Geometry: final body of the model. Coordinates: model frame, mm. Face numbers are marked on the shaded views. A direction names the side the tool comes from. Round coordinates to 2 decimals unless told otherwise and drop trailing zeros. Loops run counter-clockwise (first coordinate to the right, second up) from the corner with the lowest first, then second, coordinate; pieces in that order, holes last. Notation, with made-up numbers: (74, 15) - (129, 15) arc R21 ccw to (129, 36) - close; hole circle Ø4 at (-14, 67). An arc over 180 degrees is marked (long way). Return JSON: item names as keys, results as strings. Group by question number.
1. First-contact query: pin 1 Ø12.5 at (x, y) = (-45, 45) entering from +Z; pin 2 Ø14.5 at (x, y) = (45, 45) entering from -Z; pin 3 Ø10 at (x, y) = (-17.512, 6.5) entering from -Z; pin 4 Ø8 at (x, y) = (-18, 5.5) entering from +Z. Flat tips, straight axial feed; report the tip coordinate or a pass-through.
2. Section A-A on y = 45. Return loops of the section in (x, z), and give its area (3 significant figures).
3. Section D-D on y = 31. Return loops of the section in (x, z), and give its area (4 significant figures).
4. Material intervals for probe 1 along Y at (x, z) = (-42.5, -0.25); probe 2 along X at (y, z) = (-19, -1.5); probe 3 along X at (y, z) = (8.5, 1.25), sorted ascending.
5. Section B-B on z = 4.75. Count the separate pieces of the cut face and the enclosed holes in it, and give its area (3 significant figures).
6. Set-up query: the marked faces 1 and 2. Return all of +Z, -Z, +X, -X, +Y, -Y with unobstructed straight access to the full face (end or side cutting, diameter ignored); none if empty.
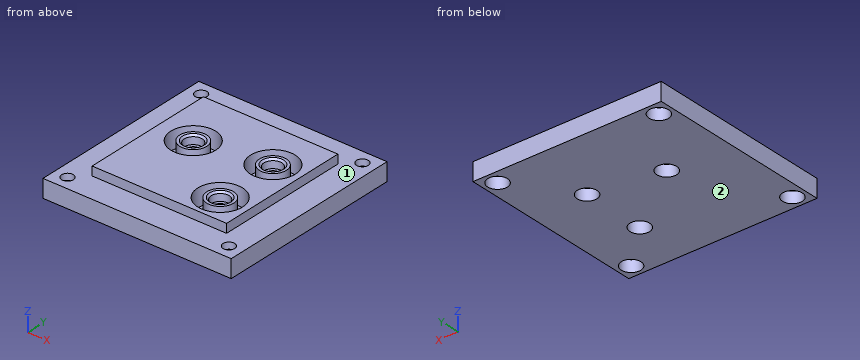
Autodesk Inventor part; units mm, degrees
ref_plane "YZ Plane" through (0, 0, 0) normal (1, 0, 0) x (0, 1, 0)
ref_plane "XZ Plane" through (0, 0, 0) normal (0, 1, 0) x (-1, 0, 0)
ref_plane "XY Plane" through (0, 0, 0) normal (0, 0, 1) x (1, 0, 0)
sketch "Skizze1" plane through (0, 0, 0) normal (0, 0, 1) x (1, 0, 0)
  line L0 (-52.5, 52.5) -> (52.5, 52.5)
  line L1 (52.5, 52.5) -> (52.5, -52.5)
  line L2 (52.5, -52.5) -> (-52.5, -52.5)
  line L3 (-52.5, -52.5) -> (-52.5, 52.5)
  line L4 (-52.5, 52.5) -> (52.5, -52.5) construction
  line L5 (52.5, 52.5) -> (-52.5, -52.5) construction
  point P0 (0, 0)
  dimension "d0" = 105
  dimension "d1" = 105
extrude "Extrusion1" add sketch "Skizze1" along normal mid plane 15
sketch "Skizze2" plane through (0, 0, -7.5) normal (0, 0, -1) x (-1, 0, 0)
  point P0 (0, 0)
  point P1 (17.512, 6.5)
  point P2 (-21.618, -22.607)
  point P3 (-21.618, 12.918)
  dimension "d4" = 21.618
  dimension "d5" = 22.607
  dimension "d6" = 12.918
  dimension "d8" = 17.512
  dimension "d16" = 6.5
hole "Bohrung1" at (21.618, -22.607, -7.5) at (21.618, 12.918, -7.5) at (-17.512, 6.5, -7.5) direction (0, 0, 1) diameter 6.6 end through all counterbore diameter 11 counterbore depth 6.4
sketch "Skizze4" plane through (0, 0, 7.5) normal (0, 0, 1) x (1, 0, 0)
  circle A0 centre (-17.512, 6.5) radius 3.3
  circle A1 centre (21.618, 12.918) radius 3.3
  circle A2 centre (21.618, -22.607) radius 3.3
  circle A3 centre (-17.512, 6.5) radius 5
  circle A4 centre (21.618, 12.918) radius 5
  circle A5 centre (21.618, -22.607) radius 5
  point P0 (0, 0)
  dimension "d24" = 10
  dimension "d25" = 10
  dimension "d26" = 10
extrude "Extrusion2" cut sketch "Skizze4" against normal blind 5 contours A0 | A1 | A2 | A3 | A4 | A5
chamfer "Fasen1" distance 1 angle 45 3 edges at (-22.512, 6.5, 7.5) (16.618, 12.918, 7.5) (16.618, -22.607, 7.5)
sketch "Skizze5" plane through (0, 0, 7.5) normal (0, 0, 1) x (1, 0, 0)
  line L0 (-37.5, 37.5) -> (37.5, 37.5)
  line L1 (37.5, 37.5) -> (37.5, -37.5)
  line L2 (37.5, -37.5) -> (-37.5, -37.5)
  line L3 (-37.5, -37.5) -> (-37.5, 37.5)
  line L4 (-37.5, 37.5) -> (37.5, -37.5) construction
  line L5 (37.5, 37.5) -> (-37.5, -37.5) construction
  line L6 (52.5, 52.5) -> (-52.5, 52.5)
  line L7 (52.5, -52.5) -> (52.5, 52.5)
  line L8 (-52.5, 52.5) -> (-52.5, -52.5)
  line L9 (-52.5, -52.5) -> (52.5, -52.5)
  point P0 (0, 0)
  dimension "d32" = 15
  dimension "d33" = 15
extrude "Extrusion3" cut sketch "Skizze5" against normal blind 5
sketch "Skizze6" plane through (0, 0, -7.5) normal (0, 0, -1) x (-1, 0, 0)
  line L0 (-52.5, -52.5) -> (52.5, -52.5)
  line L1 (52.5, -52.5) -> (52.5, 52.5)
  point P0 (0, 0)
  point P1 (45, -45)
  dimension "d36" = 7.5
  dimension "d37" = 7.5
hole "Bohrung2" at (-45, -45, -7.5) direction (0, 0, 1) diameter 6.6 end through all counterbore diameter 11 counterbore depth 6.4
pattern_circular "Runde Anordnung1" count 4 over 360 about axis through (0, 0, -10) along (0, 0, 1) of "Bohrung2"
sketch "Skizze7" plane through (0, 0, 7.5) normal (0, 0, 1) x (1, 0, 0)
  circle A0 centre (-17.512, 6.5) radius 3.3
  circle A1 centre (-17.512, 6.5) radius 7.5
  circle A2 centre (21.618, 12.918) radius 3.3
  circle A3 centre (21.618, 12.918) radius 7.5
  circle A4 centre (21.618, -22.607) radius 3.3
  circle A5 centre (21.618, -22.607) radius 7.5
  circle A6 centre (-17.512, 6.5) radius 12.5
  circle A7 centre (21.618, 12.918) radius 12.5
  circle A8 centre (21.618, -22.607) radius 5.5
  circle A9 centre (21.618, -22.607) radius 12.5
  point P0 (0, 0)
  dimension "d48" = 15
  dimension "d49" = 15
  dimension "d50" = 15
  dimension "d51" = 25
  dimension "d52" = 25
  dimension "d53" = 25
extrude "Extrusion4" cut sketch "Skizze7" against normal blind 10 contours A6 | A7 | A9
equation "\"d0\" = Breite_Magazin"
equation "\"d1\" = Tiefe_Magazin"
equation "\"d2\" = Hoehe_Bodenplatte"
equation "\"d27\" = Fuehrung_Tiefe"
equation "\"d29\" = Fase"
equation "\"d32\" = Wandstaerke"
equation "\"d33\" = Wandstaerke"
equation "\"d34\" = Fuehrung_Tiefe"
equation "\"d48\" = Feder_innen"
equation "\"d49\" = Feder_innen"
equation "\"d50\" = Feder_innen"
equation "\"d51\" = Feder_aussen"
equation "\"d52\" = Feder_aussen"
equation "\"d53\" = Feder_aussen"
equation "\"d54\" = Federfuehrung_Tiefe"
equation "\"Tiefe_Magazin\" = Breite_Magazin"
equation "\"Hoehe_Bodenplatte\" = 15"
equation "\"Fuehrung_Tiefe\" = 5"
equation "\"Fase\" = 1"
equation "\"Wandstaerke\" = 15"
equation "\"Feder_innen\" = 15"
equation "\"Feder_aussen\" = 25"
equation "\"Federfuehrung_Tiefe\" = 10"
properties part number "TS_Magazin_Grundplatte"
Taken from the geometry:
{
 "1": {"pin 1": "z = 2.5", "pin 2": "z = -7.5", "pin 3": "z = -1.1", "pin 4": "z = 6.61"},
 "2": {"outline": "(-52.5, -7.5) - (-50.5, -7.5) - (-50.5, -1.1) - (-48.3, -1.1) - (-48.3, 2.5) - (-52.5, 2.5) - close; (-41.7, -1.1) - (-39.5, -1.1) - (-39.5, -7.5) - (39.5, -7.5) - (39.5, -1.1) - (41.7, -1.1) - (41.7, 2.5) - (-41.7, 2.5) - close; (48.3, -1.1) - (50.5, -1.1) - (50.5, -7.5) - (52.5, -7.5) - (52.5, 2.5) - (48.3, 2.5) - close", "area": "862 mm2"},
 "3": {"outline": "(-52.5, -7.5) - (52.5, -7.5) - (52.5, 2.5) - (37.5, 2.5) - (37.5, 7.5) - (-37.5, 7.5) - (-37.5, 2.5) - (-52.5, 2.5) - close", "area": "1,425 mm2"},
 "4": {"probe 1": "-52.5 to -47.15, -42.85 to 42.85, 47.15 to 52.5", "probe 2": "-52.5 to 9.65, 15.04 to 17.47, 25.77 to 28.19, 33.59 to 52.5", "probe 3": "-52.5 to -29.85, -24.74 to -20.14, -14.89 to -10.28, -5.17 to 9.92, 15.56 to 27.68, 33.31 to 52.5"},
 "5": {"separate pieces": "4", "enclosed holes": "6", "area": "4,450 mm2"},
 "6": {"face 1": "+Z", "face 2": "-Z, +X, -X, +Y, -Y"}
}
